The model under review builds one solid part; all positions refer to its coordinate system, in mm. A direction names the side the tool comes from. Round coordinates to 2 decimals unless told otherwise and drop trailing zeros. Loops run counter-clockwise (first coordinate to the right, second up) from the corner with the lowest first, then second, coordinate; pieces in that order, holes last. Notation, with made-up numbers: M 78.25,54 L 97.25,54 A21 cw 97.25,68 Z; hole C -39,32 d1. An arc over 180 degrees is marked long. Answer in a Markdown table with one row per item. Add a question column.
from build123d import *

# Parameters (mm, degrees)
BOSS_EXTRUDE1_START = 50.8
BOSS_EXTRUDE1_DEPTH = 158.75


with BuildPart() as part:
    # Sketch2 → Boss-Extrude1 (new body)
    with BuildSketch(Plane(origin=(0, 0, 0), x_dir=(0, 0, -1), z_dir=(1, 0, 0)).offset(BOSS_EXTRUDE1_START)):
        with BuildLine():
            Line((223.286729101, 31.503116997), (247.278106278, 18.598154513))
            ThreePointArc((247.278106278, 18.598154513), (248.00664125, 18.315474111), (248.782155913, 18.219305384))
            Line((248.782155913, 18.219305384), (380.892090883, 18.219305384))
            ThreePointArc((380.892090883, 18.219305384), (381.606009815, 18.300611029), (382.283364565, 18.540363804))
            Line((382.283364565, 18.540363804), (406.366180194, 30.280543711))
            Line((406.366180194, 30.280543711), (407.757453877, 27.426602131))
            Line((407.757453877, 27.426602131), (383.016046062, 15.365363804))
            ThreePointArc((383.016046062, 15.365363804), (382.338691312, 15.125611029), (381.62477238, 15.044305384))
            Line((381.62477238, 15.044305384), (247.982417689, 15.044305384))
            ThreePointArc((247.982417689, 15.044305384), (247.206903026, 15.140474111), (246.478368054, 15.423154513))
            Line((246.478368054, 15.423154513), (221.782679465, 28.706966126))
            Line((221.782679465, 28.706966126), (223.286729101, 31.503116997))
        make_face()
    extrude(amount=-BOSS_EXTRUDE1_DEPTH)


solid = part.part
1. Take a section at D-D, the plane z = -233.5. State the section outline as (x, y) points.
2. Machinability: for faces 5 (the flat face through (-27.464, 21.972, -234.303)), 6 (the flat face through (-27.46, 24.33, -394.16)), which of the approach directions +Z, -Z, +X, -X, +Y, -Y give a long, thin tool a straight path to every point of the face, cutting with its end or side? Answer none if there is none.
3. To check wall thickness, follow probe 1 along Y at (x, z) = (-65, -292.5); probe 2 along Z at (x, y) = (-17, 24.25); probe 3 along Z at (x, y) = (-5.5, 28.75) (3 decimals). State the ranges of each line that lie inside material, in increasing order.
4. Mouldability with a two-part tool opening along Z and no side actions: class faces 1 (the flat face through (-107.95, 18, -315)), 2 (the flat face through (-27.464, 25.141, -235.114)), 3 (the flat face through (-27, 18.219, -314)), 4 (the flat face through (-27.5, 21.5, -395.6)) as released by +Z, released by -Z, zero draft, split by the parting line, or undercut.
5. Take a section at A-A, the plane y = 23. State the section outline as (x, z) points, and give its area (3 significant figures).
6. Take a section at B-B, the plane x = -25. State the section outline as (y, z) points (3 decimals).
7. Take a section at C-C, the plane z = -280.5. State the section outline as (x, y) points, and give its area (3 significant figures).
8. For pin 1 Ø4 at (x, y) = (-18.5, 28) entering from +Z; pin 2 Ø8 at (x, y) = (24.5, 22.5) entering from -Z; pin 3 Ø5 at (x, z) = (18, -334.5) entering from +Y, all flat-tipped, find the tip position at first contact; note any pin that passes through.
Check sheet entries:
| question | item | result |
|---|---|---|
| 1 | outline | M -107.95,22.4 L 50.8,22.4 L 50.8,26.01 L -107.95,26.01 Z |
| 2 | face 5 | +Z, +X, -X, -Y |
| 2 | face 6 | +X, -X, +Y |
| 3 | probe 1 | y = 15.04 to 18.22 |
| 3 | probe 2 | z = -401.24 to -394, -236.77 to -230.07 |
| 3 | probe 3 | z = -407.112 to -403.227, -228.405 to -221.806 |
| 4 | face 1 | zero draft |
| 4 | face 2 | undercut |
| 4 | face 3 | undercut |
| 4 | face 4 | released by -Z |
| 5 | outline | M -107.95,-398.68 L 50.8,-398.68 L 50.8,-391.43 L -107.95,-391.43 Z; M -107.95,-239.09 L 50.8,-239.09 L 50.8,-232.39 L -107.95,-232.39 Z |
| 5 | area | 2,210 mm^2 |
| 6 | outline | M 15.044,-381.625 A3.175 ccw 15.365,-383.016 L 27.427,-407.757 L 30.281,-406.366 L 18.54,-382.283 A3.175 cw 18.219,-380.892 L 18.219,-248.782 A3.175 cw 18.598,-247.278 L 31.503,-223.287 L 28.707,-221.783 L 15.423,-246.478 A3.175 ccw 15.044,-247.982 Z |
| 7 | outline | M -107.95,15.04 L 50.8,15.04 L 50.8,18.22 L -107.95,18.22 Z |
| 7 | area | 504 mm^2 |
| 8 | pin 1 | stops at z = -221.78 |
| 8 | pin 2 | stops at z = -405.86 |
| 8 | pin 3 | stops at y = 18.22 |
